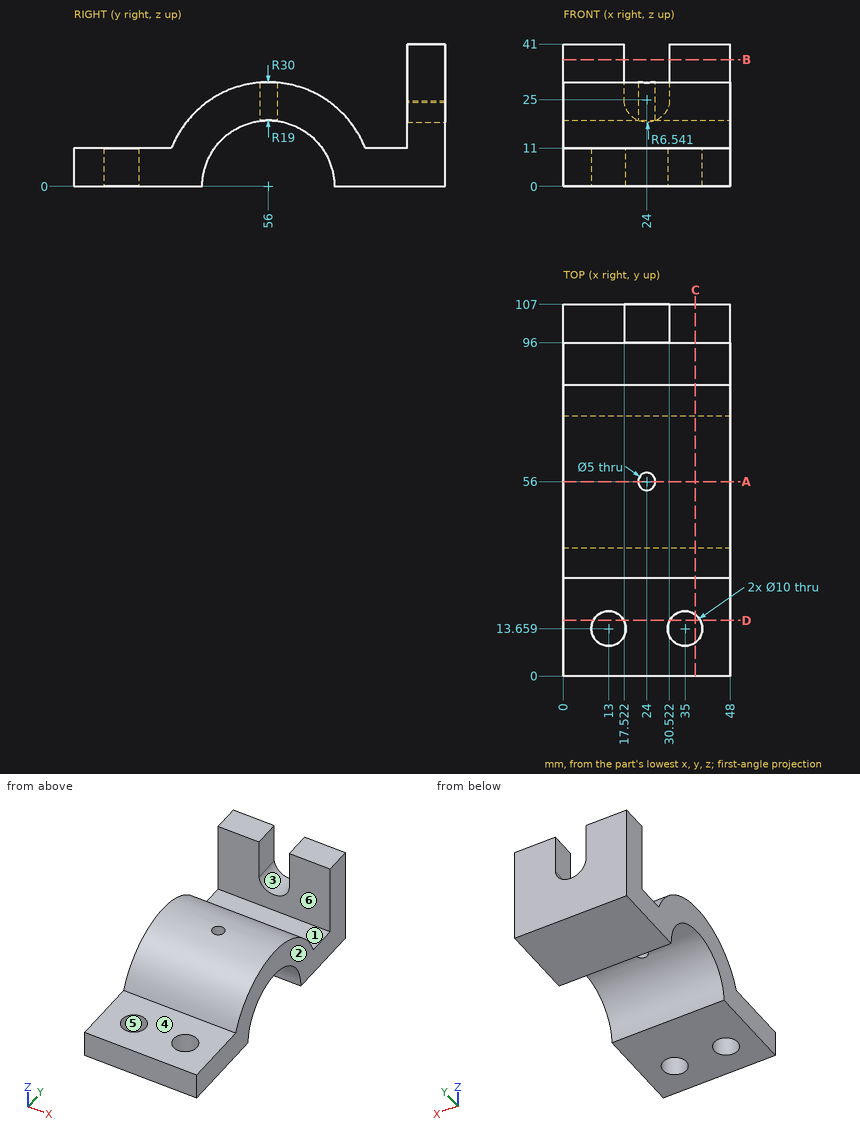
Verification items for this drawing (mm, ordinates from the low corner). A direction names the side the tool comes from. Round coordinates to 2 decimals unless told otherwise and drop trailing zeros. Write each loop counter-clockwise with the first axis right and the second up, starting at its lowest first coordinate (ties: lowest second). Pieces come first, ordered by that corner, then holes. Notation, with made-up numbers: (77, 50.25) - (128, 50.25) arc R21 cw to (128, 57.25) - close; hole circle Ø6 at (63, 70). An arc over 180 degrees is marked (long way). Answer as a JSON object with one key per item and string values. Group by question number.
Q1. Mould release check, pull along X, two halves, no side actions. Record for the marked faces 1, 2 and 3: released by +X, released by -X, zero draft, split by the parting line, or undercut.
Q2. Section check A-A, the plane y = 56. Enter the section's corners in (x, z), plus the area to 3 significant figures.
Q3. Section check C-C, the plane x = 38. Enter the section's corners in (y, z).
Q4. Thickness scan on line 1 (Y direction, x = 35, z = 3); line 2 (Y direction, x = 45, z = 13.5); line 3 (Z direction, x = 39.5, y = 23.5). Record the ranges inside material, lowest first.
Q5. Section check D-D, the plane y = 16. Enter the section's corners in (x, z).
Q6. Tool access check on the marked faces 4, 5 and 6. Record the directions out of +Z, -Z, +X, -X, +Y, -Y that give a thin tool (end or side, any length) a straight path to the whole face; none if there is none.
Q7. Section check B-B, the plane z = 36.5. Enter the section's corners in (x, y), plus the area to 3 significant figures.
Q8. Go/stop test with flat-tipped pins: pin 1 Ø8 at (x, y) = (24, 56) entering from -Z; pin 2 Ø22.5 at (x, y) = (32, 9.5) entering from +Z; pin 3 Ø5 at (x, y) = (17, 48.5) entering from -Z (1 decimal). Record where each tip stops, or that it passes through.
Found:
{
 "1": {"face 1": "zero draft", "face 2": "released by +X", "face 3": "undercut"},
 "2": {"outline": "(0, 19) - (21.5, 19) - (21.5, 30) - (0, 30) - close; (26.5, 19) - (48, 19) - (48, 30) - (26.5, 30) - close", "area": "473 mm^2"},
 "3": {"outline": "(0, 0) - (9.66, 0) - (9.66, 11) - (0, 11) - close; (17.66, 0) - (37, 0) arc R19 cw to (75, 0) - (107, 0) - (107, 41) - (96, 41) - (96, 11) - (83.91, 11) arc R30 ccw to (28.09, 11) - (17.66, 11) - close"},
 "4": {"line 1": "y = 0 to 8.66, 18.66 to 37.24, 74.76 to 107", "line 2": "y = 29.21 to 42.63, 69.37 to 82.79, 96 to 107", "line 3": "z = 0 to 11"},
 "5": {"outline": "(0, 0) - (8.58, 0) - (8.58, 11) - (0, 11) - close; (17.42, 0) - (30.58, 0) - (30.58, 11) - (17.42, 11) - close; (39.42, 0) - (48, 0) - (48, 11) - (39.42, 11) - close"},
 "6": {"face 4": "+Z, +X, -X, -Y", "face 5": "+Z, -Z", "face 6": "+Z, +X, -X"},
 "7": {"outline": "(0, 96) - (17.52, 96) - (17.52, 107) - (0, 107) - close; (30.52, 96) - (48, 96) - (48, 107) - (30.52, 107) - close", "area": "385 mm^2"},
 "8": {"pin 1": "stops at z = 18.57", "pin 2": "stops at z = 11", "pin 3": "stops at z = 16.2"}
}
